Design review of the part built by this model. Coordinates are the model's own, in mm. A direction names the side the tool comes from. Give positions to 0.01 mm unless a question says otherwise; leave off trailing zeros. Loops run counter-clockwise (first coordinate to the right, second up) from the corner with the lowest first, then second, coordinate; pieces in that order, holes last.
from build123d import *

# Parameters (mm, degrees)
F0_R     = 4.5
F1_DEPTH = 2
F2_R     = 1.99999
F3_R     = 1.35
F4_DEPTH = 3


# Not quite as in the source:
# - a fillet or chamfer is up to 0.001 mm smaller than in the source, because OpenCascade refuses the exact size


with BuildPart() as f1:
    # F0 (on Front) → F1 (new body)
    with BuildSketch(Plane.XZ):
        Circle(F0_R)
    extrude(amount=F1_DEPTH)

    # F2 (radius 2 in the source; OpenCascade refuses exactly that, so slightly less here)
    f2_edges = [f1.edges().sort_by_distance(p)[0] for p in [
        (-4.5, -2, 0),
    ]]
    fillet(f2_edges, radius=F2_R)

    # F3 (on face) → F4 (join)
    with BuildSketch(Plane(origin=(0, 0, 0), x_dir=(-1, 0, 0), z_dir=(0, 1, 0))):
        Circle(F3_R)
    extrude(amount=F4_DEPTH)


solid = f1.part
Q1. Tool access review of faces 1 (the face through (0, 3, 0)), 2 (the face through (0.29, 1.48, -1.32)): name each direction out of +Z, -Z, +X, -X, +Y, -Y from which nothing blocks a thin tool from reaching the whole face with its end or side.
Results:
face 1: +Z, -Z, +X, -X, +Y
face 2: +Y
Q2. Take a section at D-D (y = -1.15). Give the boundary of the cut face in (x, z), plus the area to 3 significant figures.
Results:
outline: circle Ø8.27 at (0, 0)
area: 53.7 mm2
Q3. Wall thickness on line 1 (Y direction, x = 1.5, z = -1.25); line 2 (X direction, y = -1.15, z = 3.5); line 3 (Z direction, x = -0.25, y = 2.45): over which ranges is each line inside the solid? List them lowest first.
Results:
line 1: y = -2 to 0
line 2: x = -2.2 to 2.2
line 3: z = -1.33 to 1.33
Q4. Insertion check: pin 1 (1 mm diameter, centred on y = 1, z = 3, fed in from -X); pin 2 (2.5 mm diameter, centred on x = -2, z = -0.5, fed in from +Y). Each pin has a flat end and moves straight along its axis. Give the tip position at first contact, or say it passes through.
Results:
pin 1: passes through
pin 2: stops at y = 3
Q5. Take a section at C-C (y = 1.3). Give the boundary of the cut face in (x, z).
Results:
outline: circle Ø2.7 at (0, 0)
